Geometry check sheet. Reference: the model listing, model coordinates, mm. Face numbers are marked on the shaded views. A direction names the side the tool comes from. Give positions to 0.01 mm unless a question says otherwise; leave off trailing zeros. Loops run counter-clockwise (first coordinate to the right, second up) from the corner with the lowest first, then second, coordinate; pieces in that order, holes last. Notation, with made-up numbers: (47, -16.5) -> (63, -16.5) arc R24 cw to (63, 12.5) -> close; hole circle Ø1 at (51.5, 41.5). An arc over 180 degrees is marked (long way). Answer in a Markdown table with one row per item. Add a question column.
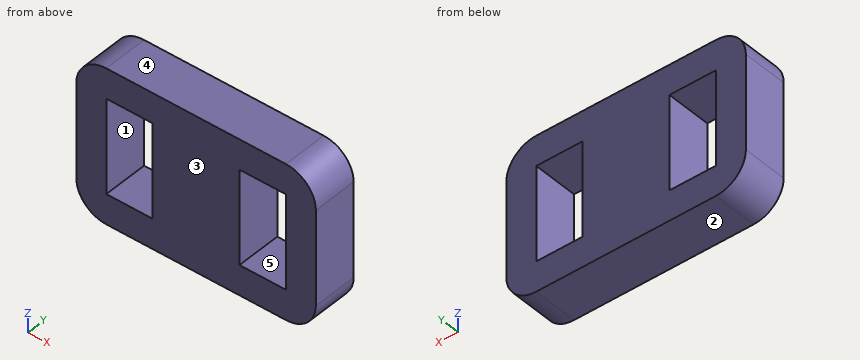
```python
from build123d import *

# Parameters (mm, degrees)
SKETCH1_W           = 3.1
SKETCH1_H           = 6.3
BOSS_EXTRUDE1_DEPTH = 3


with BuildPart() as part:
    # Sketch1 → Boss-Extrude1 (new body)
    with BuildSketch(Plane(origin=(0, 0, 0), x_dir=(1, 0, 0), z_dir=(0, 1, 0))):
        with BuildLine():
            Line((-8, 3.15), (-8, -3.15))
            ThreePointArc((-8, -3.15), (-7.414213562, -4.564213562), (-6, -5.15))
            Line((-6, -5.15), (-2.9, -5.15))
            Line((-2.9, -5.15), (6, -5.15))
            ThreePointArc((6, -5.15), (7.414213562, -4.564213562), (8, -3.15))
            Line((8, -3.15), (8, 3.15))
            ThreePointArc((8, 3.15), (7.414213562, 4.564213562), (6, 5.15))
            Line((6, 5.15), (-2.9, 5.15))
            Line((-2.9, 5.15), (-6, 5.15))
            ThreePointArc((-6, 5.15), (-7.414213562, 4.564213562), (-8, 3.15))
        make_face()
        with Locations((-4.45, 0)):
            Rectangle(SKETCH1_W, SKETCH1_H, mode=Mode.SUBTRACT)
        with Locations((4.45, 0)):
            Rectangle(SKETCH1_W, SKETCH1_H, mode=Mode.SUBTRACT)
    extrude(amount=BOSS_EXTRUDE1_DEPTH)


solid = part.part
```
1. Sectioned sample at A-A (x = -5.75). Enter the section's corners in (y, z), plus the area to 3 significant figures.
2. Gauge pin test, flat end, axial feed: pin 1 Ø5 at (x, z) = (-1, 1) entering from -Y. Record the tip position at first contact, or that the pin passes through.
3. Material ranges on L1, parallel to X at y = 2.75, z = 3; L2, parallel to Z at x = 4.5, y = 0.45; L3, parallel to Z at x = 6.25, y = 2.1, recorded low to high. Write a range as from..to.
4. Sectioned sample at C-C (y = 2.6). Enter the section's corners in (x, z).
5. Access from +Z, -Z, +X, -X, +Y, -Y to the whole of each face (thin tool, end or side, straight path). Record for the marked faces 4 and 5.
6. Sectioned sample at B-B (z = 2.75). Enter the section's corners in (x, y), plus the area to 3 significant figures.
7. Release check for a two-part mould opening along Z. For the marked faces 1, 2 and 3 record: released by +Z, released by -Z, zero draft, split by the parting line, or undercut.
Response:
| question | item | result |
|---|---|---|
| 1 | outline | (0, -5.15) -> (3, -5.15) -> (3, -3.15) -> (0, -3.15) -> close; (0, 3.15) -> (3, 3.15) -> (3, 5.15) -> (0, 5.15) -> close |
| 1 | area | 12.0 mm2 |
| 2 | pin 1 | stops at y = 0 |
| 3 | L1 | x = -8..-6, -2.9..2.9, 6..8 |
| 3 | L2 | z = -5.15..-3.15, 3.15..5.15 |
| 3 | L3 | z = -5.13..5.13 |
| 4 | outline | (-8, -3.15) arc R2 ccw to (-6, -5.15) -> (6, -5.15) arc R2 ccw to (8, -3.15) -> (8, 3.15) arc R2 ccw to (6, 5.15) -> (-6, 5.15) arc R2 ccw to (-8, 3.15) -> close; hole (-6, -3.15) -> (-2.9, -3.15) -> (-2.9, 3.15) -> (-6, 3.15) -> close; hole (2.9, -3.15) -> (6, -3.15) -> (6, 3.15) -> (2.9, 3.15) -> close |
| 5 | face 4 | +Z, +X, -X, +Y, -Y |
| 5 | face 5 | +Y, -Y |
| 6 | outline | (-8, 0) -> (-6, 0) -> (-6, 3) -> (-8, 3) -> close; (-2.9, 0) -> (2.9, 0) -> (2.9, 3) -> (-2.9, 3) -> close; (6, 0) -> (8, 0) -> (8, 3) -> (6, 3) -> close |
| 6 | area | 29.4 mm2 |
| 7 | face 1 | undercut |
| 7 | face 2 | released by -Z |
| 7 | face 3 | zero draft |
